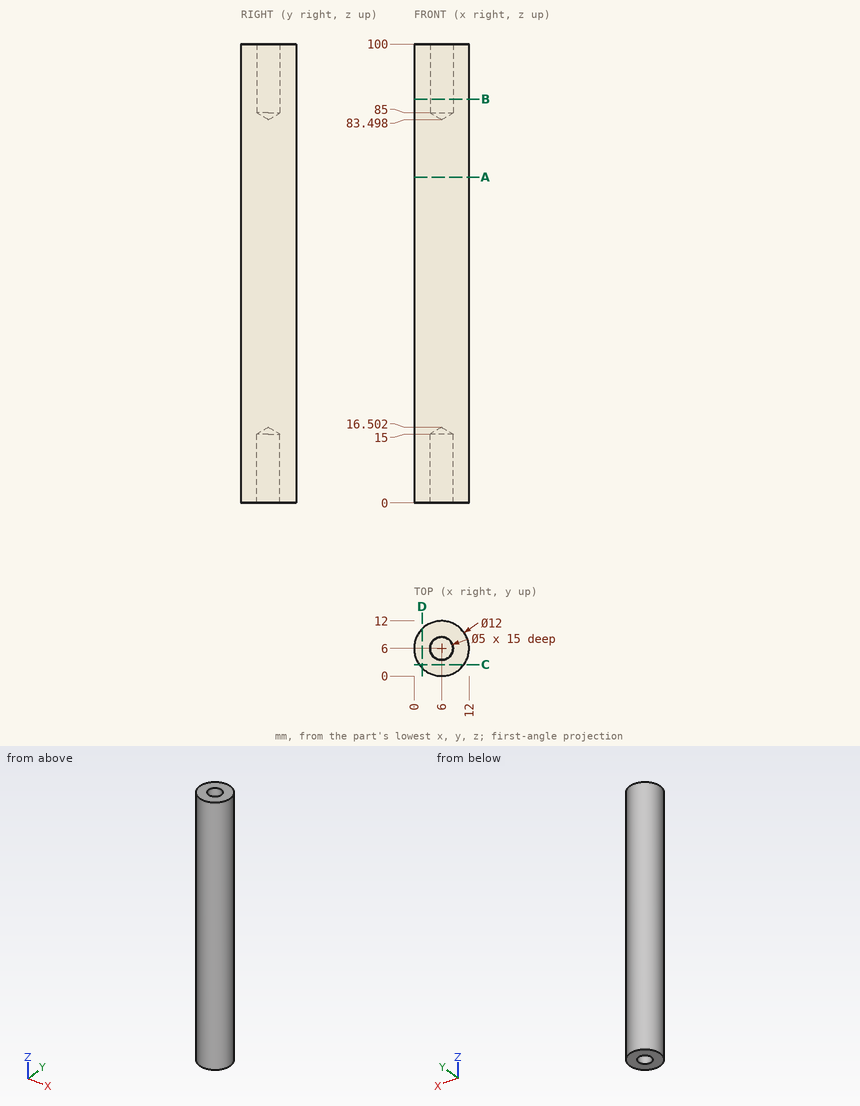
Verification items for this drawing (mm, ordinates from the low corner). Give positions to 0.01 mm unless a question says otherwise; leave off trailing zeros. Write each loop counter-clockwise with the first axis right and the second up, starting at its lowest first coordinate (ties: lowest second). Pieces come first, ordered by that corner, then holes. Notation, with made-up numbers: (-10, 39) -> (21, 39) arc R28 cw to (21, 61) -> close; hole circle Ø1 at (88.5, -15). An arc over 180 degrees is marked (long way). Use CSV: the item, a comma, the result in double quotes.
(1) Sectioned sample at C-C (y = 2.5). Record the cut outline in (x, z), plus the area to 3 significant figures.
Derived:
outline,"(1.13, 0) -> (10.87, 0) -> (10.87, 100) -> (1.13, 100) -> close"
area,"975 mm^2"
(2) Go/stop test with flat-tipped pins: pin 1 (1.5 mm diameter, centred on y = 3, z = 41, fed in from +X); pin 2 (3 mm diameter, centred on y = 3, z = 31, fed in from -X); pin 3 (1.5 mm diameter, centred on x = 7, z = 83, fed in from -Y). Record where each tip stops, or that it passes through.
Derived:
pin 1,"stops at x = 11.56"
pin 2,"stops at x = 0.19"
pin 3,"stops at y = 0.01"
(3) Sectioned sample at B-B (z = 88). Record the cut outline in (x, y).
Derived:
outline,"circle Ø12 at (6, 6); hole circle Ø5 at (6, 6)"
(4) Sectioned sample at D-D (x = 1.75). Record the cut outline in (y, z) (1 decimal), plus the area to 3 significant figures.
Derived:
outline,"(1.8, 0) -> (10.2, 0) -> (10.2, 100) -> (1.8, 100) -> close"
area,"847 mm^2"
(5) Sectioned sample at A-A (z = 71). Record the cut outline in (x, y), plus the area to 3 significant figures.
Derived:
outline,"circle Ø12 at (6, 6)"
area,"113 mm^2"
(6) Material ranges on L1, parallel to Y at x = 6, z = 94.75; L2, parallel to Y at x = 7.5, z = 7; L3, parallel to Y at x = 10.75, z = 60 (1 decimal), recorded low to high.
Derived:
L1,"y = 0 to 3.5, 8.5 to 12"
L2,"y = 0.19 to 4, 8 to 11.81"
L3,"y = 2.3 to 9.7"
